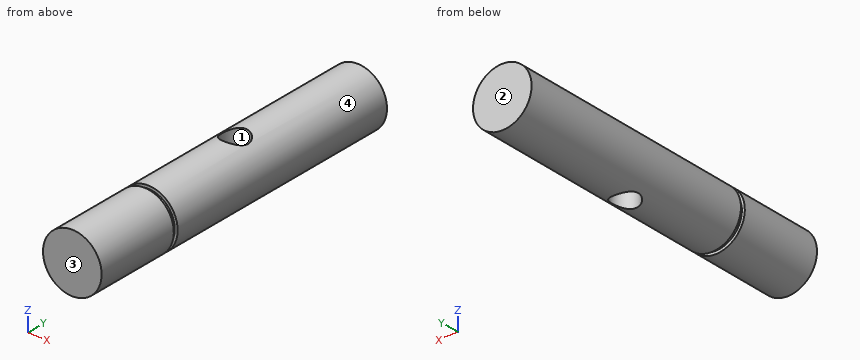
```python
from build123d import *

# Parameters (mm, degrees)
SKETCH1_R            = 5
BOSS_EXTRUDE1_DEPTH  = 59.3
CUT_EXTRUDE1_START   = -15
SKETCH2_R            = 5
SKETCH2_R_2          = 4.5
CUT_EXTRUDE1_DEPTH   = 0.8
M4_CLEARANCE_HOLE1_D = 4.5


with BuildPart() as part:
    # Sketch1 → Boss-Extrude1 (new body)
    with BuildSketch(Plane(origin=(0, 0, 0), x_dir=(1, 0, 0), z_dir=(0, 1, 0))):
        with Locations(Location((0, 0, 0), (0, 0, 90))):
            Circle(SKETCH1_R)
    extrude(amount=BOSS_EXTRUDE1_DEPTH)

    # Sketch2 → Cut-Extrude1 (cut)
    with BuildSketch(Plane.XZ.offset(CUT_EXTRUDE1_START)):
        with Locations(Location((0, 0, 0), (0, 0, 270))):
            Circle(SKETCH2_R)
        with Locations(Location((0, 0, 0), (0, 0, 270))):
            Circle(SKETCH2_R_2, mode=Mode.SUBTRACT)
    extrude(amount=-CUT_EXTRUDE1_DEPTH, mode=Mode.SUBTRACT)

    # M4 Clearance Hole1 (through all)
    with Locations(Plane.XY.offset(5)):
        with Locations((0, 33.8)):
            Hole(M4_CLEARANCE_HOLE1_D / 2)


solid = part.part
```
Work out the finished part from the listing and answer in its coordinate system (mm). Face numbers are marked on the shaded views. Round coordinates to 2 decimals unless told otherwise and drop trailing zeros. Write each loop counter-clockwise with the first axis right and the second up, starting at its lowest first coordinate (ties: lowest second). Pieces come first, ordered by that corner, then holes. Notation, with made-up numbers: (-39, 63.25) - (-24, 63.25) arc R18 ccw to (-24, 91.25) - close; hole circle Ø2 at (41.25, -8.75). An arc over 180 degrees is marked (long way). Return JSON: item names as keys, results as strings. Group by question number.
Q1. The part is cut by section D-D on z = -3.25. Write down the section's boundary in (x, y), then the cut area to 3 significant figures.
Q2. The mould has two halves that part along Y. Classify the marked faces 1, 2, 3 and 4: released by +Y, released by -Y, zero draft, split by the parting line, or undercut.
Q3. The part is cut by section B-B on z = 0. Write down the section's boundary in (x, y), then the cut area to 3 significant figures.
Q4. Each of these flat-tipped pins is pushed along its axis until it touches: pin 1 Ø3 at (x, y) = (-3, 46) entering from +Z; pin 2 Ø1 at (x, y) = (1.5, 37) entering from +Z; pin 3 Ø5 at (y, z) = (23.5, 4) entering from +X. Where does it stop, or does it pass through?
Q5. The part is cut by section A-A on x = 0. Write down the section's boundary in (y, z).
Q6. The part is cut by section C-C on y = 33.8. Write down the section's boundary in (x, z), then the cut area to 3 significant figures.
Q7. Find the intervals of material crossed by L1, parallel to Y at x = 0, z = 0; L2, parallel to X at y = 33.8, z = 0; L3, parallel to X at y = 33.8, z = 2.75, in increasing order.
Solved:
{
 "1": {"outline": "(-3.8, 0) - (3.8, 0) - (3.8, 15) - (3.11, 15) - (3.11, 15.8) - (3.8, 15.8) - (3.8, 59.3) - (-3.8, 59.3) - (-3.8, 15.8) - (-3.11, 15.8) - (-3.11, 15) - (-3.8, 15) - close; hole circle Ø4.5 at (0, 33.8)", "area": "434 mm²"},
 "2": {"face 1": "undercut", "face 2": "released by +Y", "face 3": "released by -Y", "face 4": "zero draft"},
 "3": {"outline": "(-5, 0) - (5, 0) - (5, 15) - (4.5, 15) - (4.5, 15.8) - (5, 15.8) - (5, 59.3) - (-5, 59.3) - (-5, 15.8) - (-4.5, 15.8) - (-4.5, 15) - (-5, 15) - close; hole circle Ø4.5 at (0, 33.8)", "area": "576 mm²"},
 "4": {"pin 1": "z = 4.77", "pin 2": "z = 4.9", "pin 3": "x = 4.77"},
 "5": {"outline": "(0, -5) - (15, -5) - (15, -4.5) - (15.8, -4.5) - (15.8, -5) - (31.55, -5) - (31.55, 5) - (15.8, 5) - (15.8, 4.5) - (15, 4.5) - (15, 5) - (0, 5) - close; (36.05, -5) - (59.3, -5) - (59.3, 5) - (36.05, 5) - close"},
 "6": {"outline": "(-2.25, -4.47) - (-2.25, 4.47) arc R5 ccw to start; (2.25, -4.47) arc R5 ccw to (2.25, 4.47) - close", "area": "35.1 mm²"},
 "7": {"L1": "0 to 31.55, 36.05 to 59.3", "L2": "-5 to -2.25, 2.25 to 5", "L3": "-4.18 to -2.25, 2.25 to 4.18"}
}
